from build123d import *

# Parameters (mm, degrees)
ESQUISSE1_R                                        = 50
BOSS_EXTRU_1_DEPTH                                 = 61
ESQUISSE2_R                                        = 31
ENL_V_MAT_EXTRU_1_DEPTH                            = 72
CHAMBRAGE_POUR_VIS_T_TE_RONDE_BOMB_E_M_D           = 6.6
CHAMBRAGE_POUR_VIS_T_TE_RONDE_BOMB_E_M_CBORE_D     = 13
CHAMBRAGE_POUR_VIS_T_TE_RONDE_BOMB_E_M_CBORE_DEPTH = 4.6
D_GAGEMENT_M61_D                                   = 6.6
D_GAGEMENT_M61_DEPTH                               = 5
D_GAGEMENT_M61_TIP                                 = 1.905255888
BOSS_EXTRU_2_START                                 = -61
BOSS_EXTRU_2_DEPTH                                 = 61
ESQUISSE23_R                                       = 31
ESQUISSE23_R_2                                     = 25
BOSS_EXTRU_3_DEPTH                                 = 7
ESQUISSE24_R                                       = 31
ENL_V_MAT_EXTRU_2_DEPTH                            = 3


with BuildPart() as part:
    # Esquisse1 → Boss.-Extru.1 (new body)
    with BuildSketch(Plane.XY):
        with Locations(Location((0, 0, 0), (0, 0, 180))):
            Circle(ESQUISSE1_R)
    extrude(amount=BOSS_EXTRU_1_DEPTH)

    # Esquisse2 → Enlèv. mat.-Extru.1 (cut)
    with BuildSketch(Plane(origin=(0, 0, 0), x_dir=(-1, 0, 0), z_dir=(0, 0, -1))):
        Circle(ESQUISSE2_R)
    extrude(amount=-ENL_V_MAT_EXTRU_1_DEPTH, mode=Mode.SUBTRACT)

    # Chambrage pour vis à tête ronde bombée M61 (through all)
    with Locations(Plane(origin=(0, 0, 0), x_dir=(-1, 0, 0), z_dir=(0, 0, -1))):
        with Locations((41.25, 0), (0, 41.25), (-41.25, 0), (0, -41.25)):
            CounterBoreHole(CHAMBRAGE_POUR_VIS_T_TE_RONDE_BOMB_E_M_D / 2, CHAMBRAGE_POUR_VIS_T_TE_RONDE_BOMB_E_M_CBORE_D / 2, CHAMBRAGE_POUR_VIS_T_TE_RONDE_BOMB_E_M_CBORE_DEPTH)

    # Dégagement M61
    with Locations(Plane.XY.offset(61)):
        with Locations((-23.608593004, 25.838621023), (-25.838621023, -23.608593004), (23.608593004, -25.838621023), (25.838621023, 23.608593004)):
            Hole(D_GAGEMENT_M61_D / 2, depth=D_GAGEMENT_M61_DEPTH)
            with Locations((0, 0, -(D_GAGEMENT_M61_DEPTH + D_GAGEMENT_M61_TIP / 2))):  # 120° drill point
                Cone(0, D_GAGEMENT_M61_D / 2, D_GAGEMENT_M61_TIP, mode=Mode.SUBTRACT)

    # Esquisse20 → Boss.-Extru.2 (add)
    with BuildSketch(Plane(origin=(0, 0, 0), x_dir=(-1, 0, 0), z_dir=(0, 0, -1)).offset(BOSS_EXTRU_2_START)):
        with BuildLine():
            ThreePointArc((-50, -45), (-48.535533906, -48.535533906), (-45, -50))
            Line((-45, -50), (0, -50))
            ThreePointArc((0, -50), (-35.35533911, -35.355339009), (-50, 1.43e-07))
            Line((-50, 1.43e-07), (-50, -45))
        make_face()
        with BuildLine():
            ThreePointArc((50, 0), (35.355339059, -35.355339059), (0, -50))
            Line((0, -50), (45, -50))
            ThreePointArc((45, -50), (48.535533906, -48.535533906), (50, -45))
            Line((50, -45), (50, 0))
        make_face()
        with BuildLine():
            Line((-50, 45), (-50, 1.43e-07))
            ThreePointArc((-50, 1.43e-07), (-35.355339046, 35.355339073), (-1.05e-07, 50))
            Line((-1.05e-07, 50), (-45, 50))
            ThreePointArc((-45, 50), (-48.535533906, 48.535533906), (-50, 45))
        make_face()
        with BuildLine():
            ThreePointArc((-1.05e-07, 50), (35.355339022, 35.355339097), (50, 0))
            Line((50, 0), (50, 45))
            ThreePointArc((50, 45), (48.535533906, 48.535533906), (45, 50))
            Line((45, 50), (-1.05e-07, 50))
        make_face()
    extrude(amount=BOSS_EXTRU_2_DEPTH)

    # Esquisse23 → Boss.-Extru.3 (add)
    with BuildSketch(Plane(origin=(0, 0, 0), x_dir=(-1, 0, 0), z_dir=(0, 0, -1))):
        Circle(ESQUISSE23_R)
        Circle(ESQUISSE23_R_2, mode=Mode.SUBTRACT)
    extrude(amount=-BOSS_EXTRU_3_DEPTH)

    # Esquisse24 → Enlèv. mat.-Extru.2 (cut)
    with BuildSketch(Plane(origin=(0, 0, 0), x_dir=(-1, 0, 0), z_dir=(0, 0, -1))):
        Circle(ESQUISSE24_R)
    extrude(amount=-ENL_V_MAT_EXTRU_2_DEPTH, mode=Mode.SUBTRACT)


solid = part.part
Read the model definition and answer for the solid it produces. Units are mm, in the model's axes. A direction names the side the tool comes from. Round coordinates to 2 decimals unless told otherwise and drop trailing zeros. Write each loop counter-clockwise with the first axis right and the second up, starting at its lowest first coordinate (ties: lowest second). Pieces come first, ordered by that corner, then holes. Notation, with made-up numbers: (-16.5, -5) - (39.5, -5) arc R24 cw to (39.5, 26) - close; hole circle Ø3 at (46.25, -36.75). An arc over 180 degrees is marked (long way). One line per question, with ' | ' between items. Start each with the question number.
1. For a pull along Y with two mould halves and no side action, classify faces 4 (the face through (48, 49, 31)), 5 (the face through (21, 14, 7)), 6 (the face through (50, 1, 31)), 7 (the face through (-0.43, 44.52, 33.19)) as +Y half, -Y half, draft (parallel to the pull), parting line (faces both ways), or undercut.
2. Section B-B (y = 0) is taken. Give the number of separate pieces and of enclosed holes in the cut face, and give its area (3 significant figures).
3. For faces 1 (the face through (-21.5, 22.9, 61)), 2 (the face through (-26.657, 24.575, 58.465)), 3 (the face through (2, -38, 4.6)), determine the directions among +Z, -Z, +X, -X, +Y, -Y from which every point of the face is accessible in a straight line to the end or side of a thin tool.
4. Section C-C (z = 24.5) is taken. Determine the outline of the cut face in (x, y).
5. Each of these flat-tipped pins is pushed along its axis until it touches: pin 1 (6.5 mm diameter, centred on x = 42.5, y = 1, fed in from -Z); pin 2 (21 mm diameter, centred on x = 0, y = 41.25, fed in from +Z); pin 3 (6 mm diameter, centred on x = -23.61, y = 25.84, fed in from +Z). Where does it stop, or does it pass through?
6. Section A-A (x = -41.25) is taken. Determine the outline of the cut face in (y, z).
7. Find the intervals of material crossed by probe 1 along Y at (x, z) = (0, 5); probe 2 along Y at (x, z) = (0, 47.5); probe 3 along X at (y, z) = (41.5, 36.5), in increasing order. Write a range as [from, to].
Filled in:
1) face 4: +Y half | face 5: undercut | face 6: draft | face 7: undercut
2) separate pieces: 4 | enclosed holes: 0 | area: 1,500 mm²
3) face 1: +Z, +X, -X, +Y, -Y | face 2: +Z | face 3: -Z
4) outline: (-50, -45) arc R5 ccw to (-45, -50) - (45, -50) arc R5 ccw to (50, -45) - (50, 45) arc R5 ccw to (45, 50) - (-45, 50) arc R5 ccw to (-50, 45) - close; hole circle Ø6.6 at (-41.25, 0); hole circle Ø62 at (0, 0); hole circle Ø6.6 at (0, -41.25); hole circle Ø6.6 at (0, 41.25); hole circle Ø6.6 at (41.25, 0)
5) pin 1: z = 4.6 | pin 2: z = 61 | pin 3: z = 55.83
6) outline: (-50, 0) - (-6.5, 0) - (-6.5, 4.6) - (-3.3, 4.6) - (-3.3, 61) - (-50, 61) - close; (3.3, 4.6) - (6.5, 4.6) - (6.5, 0) - (50, 0) - (50, 61) - (3.3, 61) - close
7) probe 1: [-50, -44.55], [-37.95, -25], [25, 37.95], [44.55, 50] | probe 2: [-50, -44.55], [-37.95, -31], [31, 37.95], [44.55, 50] | probe 3: [-50, -3.29], [3.29, 50]
